from build123d import *

# Parameters (mm, degrees)
F0_R     = 51.2193764732
F1_DEPTH = 71.882
F2_SIZE  = 10.16
F3_T     = -7.62


# Not quite as in the source:
# - a fillet or chamfer that OpenCascade refuses, or shapes differently, is made with other operations: its cross-section is extruded or revolved along the edge and cut away or added


with BuildPart() as f1:
    # F0 (on Right) → F1 (new body)
    with BuildSketch(Plane.YZ):
        Circle(F0_R)
    extrude(amount=F1_DEPTH)

    # F2
    f2_edges = [f1.edges().sort_by_distance(p)[0] for p in [
        (71.882, -51.219376, 0),
    ]]
    chamfer(f2_edges, length=F2_SIZE)

    # F3
    f3_openings = [f1.faces().sort_by_distance(p)[0] for p in [
        (0, 0, 0),
    ]]
    offset(amount=F3_T, openings=f3_openings)

    # F4: fillet of radius 25.4 on 1 edges, made by hand

    # F4_s1 → F4_t2 (revolve, cut)
    with BuildSketch(Plane.XY):
        with BuildLine():
            ThreePointArc((18.1392282085, 51.2193764732), (8.3018505091, 49.2370193947), (0, 43.5993764732))
            Line((0, 43.5993764732), (0, 51.2193764732))
            Line((0, 51.2193764732), (18.1392282085, 51.2193764732))
        make_face()
    revolve(axis=Axis((0, 0, 0), (1, 0, 0)), mode=Mode.SUBTRACT)


solid = f1.part
Source: CAD feature listing. Evaluate the final solid. Frame: model axes, mm. A direction names the side the tool comes from. Coordinates: 2 decimals unless noted, no trailing zeros. Order: outer loops, then holes, each group sorted by start corner. A loop starts at its lowest first (then second) coordinate and runs counter-clockwise, first axis right, second up.
Item 1: Cut plane A-A (z = 0). Return loops of the section in (x, y).
Output values:
outline: (0, -43.6) arc R25.4 ccw to (18.14, -51.22) - (61.72, -51.22) - (71.88, -41.06) - (71.88, 41.06) - (61.72, 51.22) - (18.14, 51.22) arc R25.4 ccw to (0, 43.6) - (58.57, 43.6) - (64.26, 37.9) - (64.26, -37.9) - (58.57, -43.6) - close
Item 2: Cut plane D-D (x = 67.5). Return loops of the section in (y, z).
Output values:
outline: circle Ø90.88 at (0, 0)
Item 3: Pull-direction query (Y, two-part tool) for faces 1 (the face through (64.262, -1, 1)), 2 (the face through (39.626, -11.103, -50.001)), 3 (the face through (71.882, -1, 1)); classes: pulls with the +Y half, pulls with the -Y half, needs draft (parallel to the pull), parting line crosses it, or undercut.
Output values:
face 1: undercut
face 2: parting line crosses it
face 3: needs draft
Item 4: Set-up query: faces 4 (the face through (28.873, -9.451, -42.563)), 5 (the face through (71.39, 39.63, 12.48)). Return all of +Z, -Z, +X, -X, +Y, -Y with unobstructed straight access to the full face (end or side cutting, diameter ignored); none if empty.
Output values:
face 4: -X
face 5: +X
Item 5: First-contact query: P1, Ø8, axis at y = 8, z = -12.5, coming from the -X side; P2, Ø1, axis at x = 27, z = 18.5, coming from the -Y side; P3, Ø3, axis at x = 9, z = -21.5, coming from the -Y side. Flat tips, straight axial feed; report the tip coordinate or a pass-through.
Output values:
P1: stops at x = 64.26
P2: stops at y = -47.95
P3: stops at y = -45.53
Item 6: Cut plane B-B (x = 48). Return loops of the section in (y, z), plus the area to 3 significant figures.
Output values:
outline: circle Ø102.44 at (0, 0); hole circle Ø87.2 at (0, 0)
area: 2,270 mm2
Item 7: Material intervals for line 1 (Z direction, x = 25, y = 0); line 2 (X direction, y = 5, z = 4.5); line 3 (Z direction, x = 48.5, y = 13), sorted ascending.
Output values:
line 1: z = -51.22 to -43.6, 43.6 to 51.22
line 2: x = 64.26 to 71.88
line 3: z = -49.54 to -41.62, 41.62 to 49.54
